Source: three-view drawing plus pictorial views. Frame: mm from the lowest corner of the part. Coordinates: 2 decimals unless noted, no trailing zeros. Order: outer loops, then holes, each group sorted by start corner. A loop starts at its lowest first (then second) coordinate and runs counter-clockwise, first axis right, second up. Notation, with made-up numbers: M -34.75,-15.75 L -8.75,-15.75 A21 cw -8.75,-6.75 Z; hole C 4.25,-2 d5. An arc over 180 degrees is marked long. Use CSV: the item, a comma, the result in double quotes. Start each with the question number.
Q1. Section query B-B, the plane z = 0.65. State how many separate pieces and enclosed holes the cut face has, and give its area (3 significant figures).
Q2. Section query A-A, the plane y = 12.7. Output: boundary loops of the cut face in (x, z) (1 decimal), and give its area (3 significant figures).
Q3. Section query C-C, the plane x = 12.7. Output: boundary loops of the cut face in (y, z) (1 decimal).
Q4. Ray query, probe 1 along Y at (x, z) = (63.5, 1.6) (1 decimal); probe 2 along X at (y, z) = (45.5, 2.15) (1 decimal); probe 3 along X at (y, z) = (44, 1.4) (1 decimal). Return the intervals inside material, ascending.
Q5. Section query D-D, the plane y = 43.5. Output: boundary loops of the cut face in (x, z) (1 decimal).
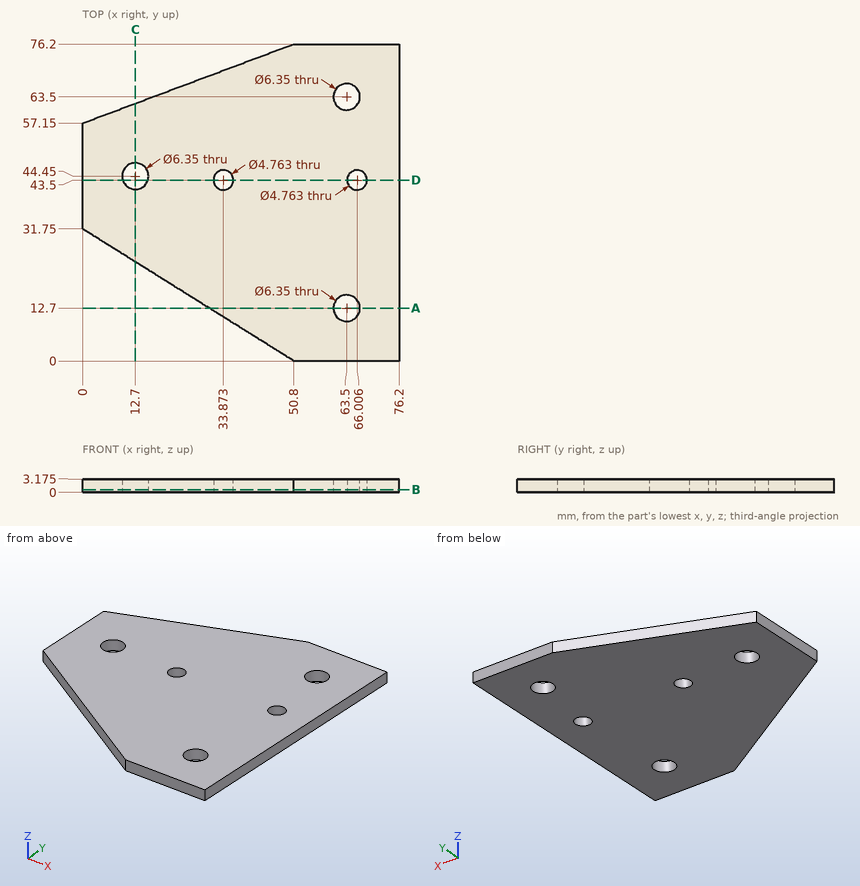
Responses:
1,separate pieces,"1"
1,enclosed holes,"5"
1,area,"4,390 mm²"
2,outline,"M 30.5,0 L 60.3,0 L 60.3,3.2 L 30.5,3.2 Z; M 66.7,0 L 76.2,0 L 76.2,3.2 L 66.7,3.2 Z"
2,area,"125 mm²"
3,outline,"M 23.8,0 L 41.3,0 L 41.3,3.2 L 23.8,3.2 Z; M 47.6,0 L 61.9,0 L 61.9,3.2 L 47.6,3.2 Z"
4,probe 1,"y = 0 to 9.5, 15.9 to 60.3, 66.7 to 76.2"
4,probe 2,"x = 0 to 9.7, 15.7 to 32.6, 35.2 to 64.7, 67.3 to 76.2"
4,probe 3,"x = 0 to 9.6, 15.8 to 31.5, 36.2 to 63.7, 68.3 to 76.2"
5,outline,"M 0,0 L 9.7,0 L 9.7,3.2 L 0,3.2 Z; M 15.7,0 L 31.5,0 L 31.5,3.2 L 15.7,3.2 Z; M 36.3,0 L 63.6,0 L 63.6,3.2 L 36.3,3.2 Z; M 68.4,0 L 76.2,0 L 76.2,3.2 L 68.4,3.2 Z"
